Autodesk Inventor part; units mm, degrees
ref_plane "YZ Plane" through (0, 0, 0) normal (1, 0, 0) x (0, 1, 0)
ref_plane "XZ Plane" through (0, 0, 0) normal (0, 1, 0) x (-1, 0, 0)
ref_plane "XY Plane" through (0, 0, 0) normal (0, 0, 1) x (1, 0, 0)
sketch "Sketch1" plane through (0, 0, 0) normal (0, 1, 0) x (-1, 0, 0)
  line L0 (-40, -100) -> (40, -100)
  line L1 (40, -100) -> (40, 100)
  line L2 (40, 100) -> (-40, 100)
  line L3 (-40, 100) -> (-40, -100)
  line L4 (-40, -100) -> (40, 100) construction
  line L5 (40, -100) -> (-40, 100) construction
  point P0 (0, 0)
  dimension "d0" = 80
  dimension "d1" = 200
extrude "Extrusion1" add sketch "Sketch1" along normal blind 5
sketch "Sketch2" plane through (0, 5, 0) normal (0, 1, 0) x (1, 0, 0)
  line L0 (-40, 100) -> (-40, -100)
  line L1 (-40, -100) -> (40, -100)
  line L2 (40, -100) -> (40, 100)
  line L3 (40, 100) -> (-40, 100)
  line L4 (37, 97) -> (-37, 97)
  line L5 (-37, 97) -> (-37, -97)
  line L6 (-37, -97) -> (37, -97)
  line L7 (37, -97) -> (37, 97)
  line L8 (37, 97) -> (-37, -97) construction
  line L9 (-37, 97) -> (37, -97) construction
  line L10 (34, 94) -> (-34, 94)
  line L11 (-34, 94) -> (-34, -94)
  line L12 (-34, -94) -> (34, -94)
  line L13 (34, -94) -> (34, 94)
  line L14 (34, 94) -> (-34, -94) construction
  line L15 (-34, 94) -> (34, -94) construction
  point P0 (0, 0)
  dimension "d4" = 3
  dimension "d5" = 3
  dimension "d6" = 3
  dimension "d7" = 3
extrude "Extrusion2" add sketch "Sketch2" along normal blind 25 contours L7 L6 L5 L4
fillet "Fillet1" radius 2 4 edges at (-37, 17.5, 97) (37, 17.5, 97) (37, 17.5, -97) (-37, 17.5, -97)
fillet "Fillet2" radius 2 4 edges at (-40, 2.5, 100) (40, 2.5, 100) (40, 2.5, -100) (-40, 2.5, -100)
sketch "Sketch3" plane through (37, 5, 95) normal (1, 0, 0) x (0, 0, -1)
  line L0 (190, 25) -> (190, 0)
  line L1 (0, 25) -> (190, 25)
  line L2 (0, 0) -> (0, 25)
  line L3 (190, 0) -> (0, 0)
  line L4 (5, 22.5) -> (185, 22.5)
  line L5 (185, 22.5) -> (185, 2.5)
  line L6 (185, 2.5) -> (5, 2.5)
  line L7 (5, 2.5) -> (5, 22.5)
  line L8 (-2, 25) -> (-2, 0)
  line L9 (192, 0) -> (192, 25)
  line L10 (195, -5) -> (195, 0)
  line L11 (-5, 0) -> (-5, -5)
  point P0 (95, -5)
  point P1 (185, 12.5)
  point P2 (-2, 12.5)
  dimension "d33" = 20
  dimension "d34" = 10
  dimension "d35" = 10
  dimension "d36" = 10
extrude "Extrusion3" add sketch "Sketch3" along normal blind 6 contours L4 L5 L6 L7
sketch "Sketch4" plane through (37, 7.5, -90) normal (0, 0, -1) x (-1, 0, 0)
  line L0 (0, 20) -> (0, 0)
  line L1 (0, 20) -> (-6, 20)
  line L2 (-6, 0) -> (-6, 20)
  line L3 (0, 0) -> (-6, 0)
  line L4 (-6, 0) -> (-6, 20)
  line L5 (-6, 12.5) -> (-3, 12.5)
  line L6 (-3, 12.5) -> (-3, 7.5)
  line L7 (-3, 7.5) -> (-6, 7.5)
  line L8 (-6, 7.5) -> (-6, 12.5)
  line L9 (0, -2.5) -> (0, 22.5)
  line L10 (0, 15) -> (-3, 15)
  line L11 (-3, 15) -> (-3, 5)
  line L12 (-3, 5) -> (0, 5)
  line L13 (0, 5) -> (0, 15)
  point P0 (37, -7.5)
  point P1 (-4.5, 12.5)
  point P2 (-6, 7.5)
  point P3 (-3, 7.5)
  point P4 (0, 5)
  point P5 (-3, 12.5)
  point P6 (-1.5, 5)
  dimension "d19" = 3
  dimension "d22" = 5
  dimension "d23" = 5
  dimension "d37" = 2.5
  dimension "d38" = 2.5
extrude "Extrusion4" cut sketch "Sketch4" against normal blind 170 contours L0 L12 L11 L6 L10 | L5 L6 L7 L2
fillet "Fillet3" radius 2 3 edges at (43, 17.5, 90) (43, 11.25, -90) (43, 23.75, -90)
sketch "Sketch5" plane through (-37, 5, -95) normal (-1, 0, 0) x (0, 0, 1)
  line L0 (0, 25) -> (190, 25)
  line L1 (-2, 25) -> (-2, 0)
  line L2 (192, 0) -> (192, 25)
  line L3 (5, 17.5) -> (175, 17.5)
  line L4 (175, 17.5) -> (175, 7.5)
  line L5 (175, 7.5) -> (5, 7.5)
  line L6 (5, 7.5) -> (5, 17.5)
  line L7 (-5, 0) -> (-5, -5)
  line L8 (195, -5) -> (195, 0)
  point P0 (95, -5)
  point P1 (192, 12.5)
  dimension "d28" = 10
  dimension "d39" = 10
  dimension "d40" = 20
  dimension "d41" = 5
extrude "Extrusion5" add sketch "Sketch5" along normal blind 6
sketch "Sketch6" plane through (-37, 12.5, 80) normal (0, 0, 1) x (1, 0, 0)
  line L0 (0, 10) -> (0, 0)
  line L1 (0, 10) -> (-6, 10)
  line L2 (-6, 0) -> (-6, 10)
  line L3 (0, 0) -> (-6, 0)
  line L4 (0, 10) -> (-3, 10)
  line L5 (-3, 10) -> (-3, 7.5)
  line L6 (-3, 7.5) -> (0, 7.5)
  line L7 (0, 7.5) -> (0, 10)
  line L8 (0, 0) -> (-3, 0)
  line L9 (-3, 0) -> (-3, 2.5)
  line L10 (-3, 2.5) -> (0, 2.5)
  line L11 (0, 2.5) -> (0, 0)
  point P0 (37, -12.5)
  point P1 (0, 2.5)
  point P2 (-3, 0)
  point P3 (0, 7.5)
  point P4 (-3, 10)
  dimension "d44" = 3
  dimension "d45" = 2.5
  dimension "d46" = 3
  dimension "d47" = 2.5
extrude "Extrusion6" cut sketch "Sketch6" against normal up to surface (170 mm away) contours L0 L6 L5 L1 | L0 L3 L9 L10
fillet "Fillet4" radius 1 18 edges at (-43, 22.5, -5) (-40, 22.5, -5) (-43, 12.5, -5) (-40, 12.5, -5) (-43, 17.5, 80) (-40, 21.25, 80) (-41.5, 22.5, 80) (-41.5, 12.5, 80) (-40, 13.75, 80) (-40, 13.75, -90) (-43, 17.5, -90) (-40, 21.25, -90) (-41.5, 22.5, -90) (-41.5, 12.5, -90) (-38.5, 20, -90) (-38.5, 15, -90) (-38.5, 15, 80) (-38.5, 20, 80)
properties part number "module_command"
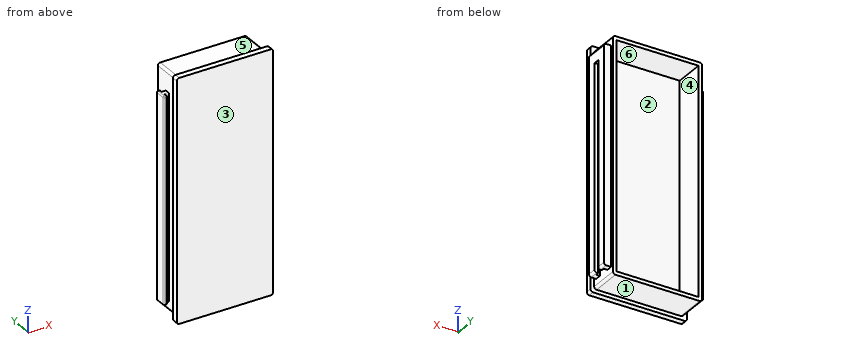
CAD build for the part. Positions are in the model's coordinates, mm. Face numbers are marked on the shaded views. A direction names the side the tool comes from. Round coordinates to 2 decimals unless told otherwise and drop trailing zeros. Order: outer loops, then holes, each group sorted by start corner. A loop starts at its lowest first (then second) coordinate and runs counter-clockwise, first axis right, second up.
Q1. Wall check: L1, parallel to Z at x = -20, y = 15.75; L2, parallel to X at y = 22.75, z = -15; L3, parallel to X at y = 19.5, z = -1.5. Give the ranges that are in metal, low to high.
Q2. Slice it at A-A (y = 24.75). Write the cut outline in (x, z).
Q3. Which spindle directions (+Z, -Z, +X, -X, +Y, -Y) get a long thin tool onto all of the face, cutting with end or side? Do the marked faces 1, 2 and 3. Say none if no direction does.
Q4. Slice it at B-B (x = 23). Write the cut outline in (y, z), and give its area (3 significant figures).
Q5. Two-plate mould, pull along X, no slides. Class the marked faces 4, 5 and 6: pulls with the +X half, pulls with the -X half, needs draft (parallel to the pull), parting line crosses it, or undercut.
Q6. Drop flat-ended pins along their axis: pin 1 (3 mm diameter, centred on x = 39.5, y = 16.5, fed in from -Z); pin 2 (1 mm diameter, centred on x = -13, y = 19.5, fed in from -Z); pin 3 (1 mm diameter, centred on x = -11.5, z = -33, fed in from +Y). Give the stop position or say it passes through.
Results below:
1. L1: z = -97 to -94, 94 to 97
1. L2: x = -37 to -34, 34 to 43
1. L3: x = -43 to -34, 34 to 37
2. outline: (-37, -95) arc R2 ccw to (-35, -97) - (35, -97) arc R2 ccw to (37, -95) - (37, -90) - (41, -90) arc R2 ccw to (43, -88) - (43, 88) arc R2 ccw to (41, 90) - (37, 90) - (37, 95) arc R2 ccw to (35, 97) - (-35, 97) arc R2 ccw to (-37, 95) - close; hole (-34, -94) - (34, -94) - (34, 94) - (-34, 94) - close
3. face 1: -Z, +X, -X, +Y
3. face 2: +Y
3. face 3: +Z, -Z, +X, -X, -Y
4. outline: (0, -100) - (5, -100) - (5, -97) - (30, -97) - (30, -94) - (5, -94) - (5, 94) - (30, 94) - (30, 97) - (5, 97) - (5, 100) - (0, 100) - close
4. area: 1,150 mm2
5. face 4: undercut
5. face 5: needs draft
5. face 6: undercut
6. pin 1: stops at z = 80
6. pin 2: stops at z = -97
6. pin 3: stops at y = 5
